from build123d import *

# Parameters (mm, degrees)
ESBO_O1_W                = 46.4
ESBO_O1_H                = 22
ESBO_O1_R                = 0.95
RESSALTO_EXTRUS_O1_DEPTH = 4.5
ESBO_O2_W                = 46.4
ESBO_O2_H                = 22
RESSALTO_EXTRUS_O2_DEPTH = 0.5
ESBO_O4_R                = 1.05
CORTE_EXTRUS_O2_DEPTH    = 10.5
ESBO_O8_R                = 2
CORTE_EXTRUS_O3_DEPTH    = 3
RESSALTO_EXTRUS_O3_DEPTH = 0.5
ESBO_O11_R               = 0.75
CORTE_EXTRUS_O5_DEPTH    = 10
ESBO_O12_W               = 40.744
ESBO_O12_H               = 10
CORTE_EXTRUS_O6_DEPTH    = 4.5


with BuildPart() as part:
    # Esboço1 → Ressalto-extrusão1 (new body)
    with BuildSketch(Plane(origin=(0, 0, 0), x_dir=(1, 0, 0), z_dir=(0, 1, 0))):
        Rectangle(ESBO_O1_W, ESBO_O1_H)
        with Locations(Location((20.372, -8, 0), (0, 0, 270))):
            Circle(ESBO_O1_R, mode=Mode.SUBTRACT)
        with Locations(Location((-20.372, 8, 0), (0, 0, 270))):
            Circle(ESBO_O1_R, mode=Mode.SUBTRACT)
        Polygon((-21.2, 5), (-17.544, 5), (-17.544, 8.05), (17.544, 8.05), (17.544, 5), (21.2, 5), (21.2, -5), (17.544, -5), (17.544, -8.15), (-17.544, -8.15), (-17.544, -5), (-21.2, -5), align=None, mode=Mode.SUBTRACT)
    extrude(amount=RESSALTO_EXTRUS_O1_DEPTH)

    # Esboço2 → Ressalto-extrusão2 (add)
    with BuildSketch(Plane.XZ):
        Rectangle(ESBO_O2_W, ESBO_O2_H)
    extrude(amount=RESSALTO_EXTRUS_O2_DEPTH)

    # Esboço4 → Corte-extrusão2 (cut)
    with BuildSketch(Plane(origin=(0, 0, 0), x_dir=(1, 0, 0), z_dir=(0, 1, 0))):
        with Locations(Location((20.372, -8, 0), (0, 0, 270))):
            Circle(ESBO_O4_R)
        with Locations(Location((-20.372, 8, 0), (0, 0, 270))):
            Circle(ESBO_O4_R)
    extrude(amount=-CORTE_EXTRUS_O2_DEPTH, mode=Mode.SUBTRACT)

    # Esboço8 → Corte-extrusão3 (cut)
    with BuildSketch(Plane(origin=(0, -0.5, 0), x_dir=(1, 0, 0), z_dir=(0, 1, 0))):
        with Locations(Location((20.372, -8, 0), (0, 0, 270))):
            Circle(ESBO_O8_R)
        with Locations(Location((-20.372, 8.05, 0), (0, 0, 270))):
            Circle(ESBO_O8_R)
    extrude(amount=CORTE_EXTRUS_O3_DEPTH, mode=Mode.SUBTRACT)

    # Esboço10 → Ressalto-extrusão3 (add, symmetric)
    with BuildSketch(Plane(origin=(0, 0, 0), x_dir=(1, 0, 0), z_dir=(0, 1, 0))):
        with BuildLine():
            Line((-23.2, 11), (-26.7, 11))
            ThreePointArc((-26.7, 11), (-27.053553391, 10.853553391), (-27.2, 10.5))
            Line((-27.2, 10.5), (-27.2, 5.5))
            ThreePointArc((-27.2, 5.5), (-27.053553391, 5.146446609), (-26.7, 5))
            Line((-26.7, 5), (-23.2, 5))
            Line((-23.2, 5), (-23.2, 11))
        make_face()
        with BuildLine():
            Line((-23.2, -11), (-26.7, -11))
            ThreePointArc((-26.7, -11), (-27.053553391, -10.853553391), (-27.2, -10.5))
            Line((-27.2, -10.5), (-27.2, -5.5))
            ThreePointArc((-27.2, -5.5), (-27.053553391, -5.146446609), (-26.7, -5))
            Line((-26.7, -5), (-23.2, -5))
            Line((-23.2, -5), (-23.2, -11))
        make_face()
        with BuildLine():
            Line((23.2, 11), (26.7, 11))
            ThreePointArc((26.7, 11), (27.053553391, 10.853553391), (27.2, 10.5))
            Line((27.2, 10.5), (27.2, 5.5))
            ThreePointArc((27.2, 5.5), (27.053553391, 5.146446609), (26.7, 5))
            Line((26.7, 5), (23.2, 5))
            Line((23.2, 5), (23.2, 11))
        make_face()
        with BuildLine():
            Line((23.2, -11), (26.7, -11))
            ThreePointArc((26.7, -11), (27.053553391, -10.853553391), (27.2, -10.5))
            Line((27.2, -10.5), (27.2, -5.5))
            ThreePointArc((27.2, -5.5), (27.053553391, -5.146446609), (26.7, -5))
            Line((26.7, -5), (23.2, -5))
            Line((23.2, -5), (23.2, -11))
        make_face()
    extrude(amount=RESSALTO_EXTRUS_O3_DEPTH, both=True)

    # Esboço11 → Corte-extrusão5 (cut)
    with BuildSketch(Plane(origin=(0, 0.5, 0), x_dir=(1, 0, 0), z_dir=(0, 1, 0))):
        with Locations(Location((-25.2, 8, 0), (0, 0, 270))):
            Circle(ESBO_O11_R)
        with Locations(Location((-25.2, -8, 0), (0, 0, 270))):
            Circle(ESBO_O11_R)
        with Locations(Location((25.2, -8, 0), (0, 0, 270))):
            Circle(ESBO_O11_R)
        with Locations(Location((25.2, 8, 0), (0, 0, 270))):
            Circle(ESBO_O11_R)
    extrude(amount=-CORTE_EXTRUS_O5_DEPTH, mode=Mode.SUBTRACT)

    # Esboço12 → Corte-extrusão6 (cut)
    with BuildSketch(Plane(origin=(0, 4.5, 0), x_dir=(1, 0, 0), z_dir=(0, 1, 0))):
        with Locations((-2.828, 0)):
            Rectangle(ESBO_O12_W, ESBO_O12_H)
    extrude(amount=-CORTE_EXTRUS_O6_DEPTH, mode=Mode.SUBTRACT)


solid = part.part
Check sheet for the modelled part. Datum: model origin and axes. Units: mm. A direction names the side the tool comes from. Give positions to 0.01 mm unless a question says otherwise; leave off trailing zeros. Write each loop counter-clockwise with the first axis right and the second up, starting at its lowest first coordinate (ties: lowest second). Pieces come first, ordered by that corner, then holes. Notation, with made-up numbers: (-28, -25) -> (-12, -25) arc R27 cw to (-12, -3) -> close; hole circle Ø9 at (-14.75, 9.5). An arc over 180 degrees is marked (long way). Write item = value, one per line.
Item 1: Sectioned sample at D-D on y = 4. Record the boundary of the cut face in (x, z).
Output:
outline = (-23.2, -11) -> (23.2, -11) -> (23.2, 11) -> (-23.2, 11) -> (-23.2, 5) -> (-17.54, 5) -> (-17.54, 8.15) -> (17.54, 8.15) -> (17.54, 5) -> (21.2, 5) -> (21.2, -5) -> (17.54, -5) -> (17.54, -8.05) -> (-17.54, -8.05) -> (-17.54, -5) -> (-23.2, -5) -> close; hole circle Ø1.9 at (-20.37, -8); hole circle Ø1.9 at (20.37, 8)
Item 2: Scan lines: probe 1 along X at (y, z) = (0.25, 8); probe 2 along X at (y, z) = (3.9, -8); probe 3 along X at (y, z) = (3.3, -7.5). Record each from-to range of solid material in increasing order. Write a range as from..to.
Output:
probe_1 = -27.2..-25.95, -24.45..-17.54, 17.54..18.37, 22.37..24.45, 25.95..27.2
probe_2 = -23.2..-21.32, -19.42..-17.54, 17.54..23.2
probe_3 = -23.2..-21.18, -19.56..-17.54, 17.54..23.2
Item 3: Sectioned sample at C-C on z = 3.5. Record the boundary of the cut face in (x, y), and give its area (3 significant figures).
Output:
outline = (-23.2, -0.5) -> (23.2, -0.5) -> (23.2, 4.5) -> (21.2, 4.5) -> (21.2, 0) -> (-23.2, 0) -> close
area = 32.2 mm^2
Item 4: Tool access check on faces 4 (the flat face through (17.544, 2, -7)), 5 (the flat face through (-26, 0.5, 9)), 6 (the cylindrical face through (25.944, 0.007, -8.098)), 7 (the flat face through (19, 2, -5)), 8 (the flat face through (25, 0, 5)). Record the directions out of +Z, -Z, +X, -X, +Y, -Y that give a thin tool (end or side, any length) a straight path to the whole face; none if there is none.
Output:
face_4 = +Y
face_5 = +Z, -Z, -X, +Y
face_6 = +Y, -Y
face_7 = -X, +Y
face_8 = +X, +Y, -Y
Item 5: Gauge pin test, flat ends, axial feed: pin 1 (1 mm diameter, centred on y = 3, z = -1, fed in from -X); pin 2 (1.2 mm diameter, centred on y = 2.5, z = -7.5, fed in from -X); pin 3 (1.2 mm diameter, centred on x = 25, z = -9, fed in from +Y). Record the tip position at first contact, or that the pin passes through.
Output:
pin_1 = 21.2
pin_2 = -23.2
pin_3 = 0.5
Item 6: Release check for a two-part mould opening along X. For faces 1 (the flat face through (-23.2, 3, -8)), 2 (the cylindrical face through (-24.69, 0.01, 7.45)), 3 (the flat face through (-21, 2, -5)) record: +X half, -X half, draft (parallel to the pull), parting line (faces both ways), or undercut.
Output:
face_1 = -X half
face_2 = undercut
face_3 = draft
Item 7: Sectioned sample at B-B on x = -10. Record the boundary of the cut face in (y, z).
Output:
outline = (-0.5, -11) -> (4.5, -11) -> (4.5, -8.05) -> (0, -8.05) -> (0, 8.15) -> (4.5, 8.15) -> (4.5, 11) -> (-0.5, 11) -> close
Item 8: Sectioned sample at A-A on x = -25.2. Record the boundary of the cut face in (y, z), and give its area (3 significant figures).
Output:
outline = (-0.5, -11) -> (0.5, -11) -> (0.5, -8.75) -> (-0.5, -8.75) -> close; (-0.5, -7.25) -> (0.5, -7.25) -> (0.5, -5) -> (-0.5, -5) -> close; (-0.5, 5) -> (0.5, 5) -> (0.5, 7.25) -> (-0.5, 7.25) -> close; (-0.5, 8.75) -> (0.5, 8.75) -> (0.5, 11) -> (-0.5, 11) -> close
area = 9.00 mm^2
